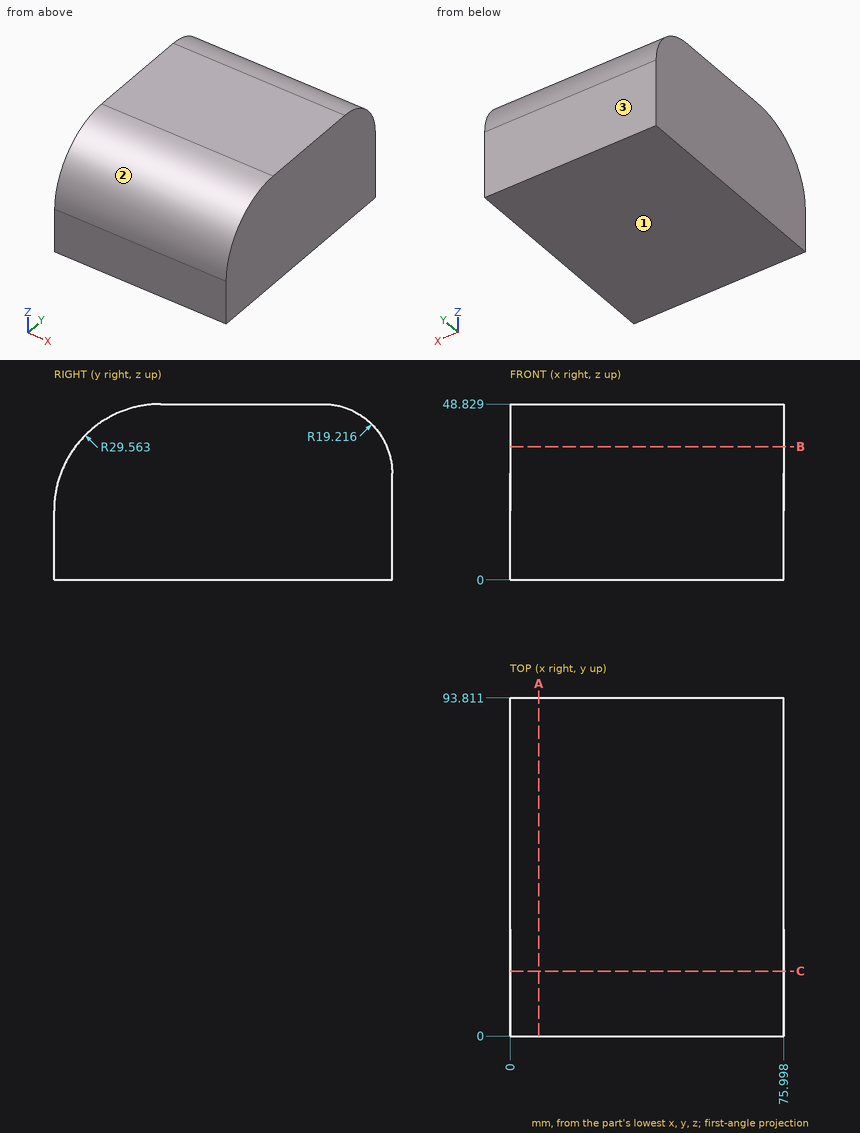
Input: dimensioned drawing with shaded views. Units: mm. Origin: part minimum x, y, z. Give positions to 0.01 mm unless a question says otherwise; leave off trailing zeros. Write each loop counter-clockwise with the first axis right and the second up, starting at its lowest first coordinate (ties: lowest second). Pieces come first, ordered by that corner, then holes. Notation, with made-up numbers: M 85,-28.75 L 133,-28.75 A7 cw 133,-22.75 Z; hole C 74.5,14.25 d4. An arc over 180 degrees is marked long. Write item = value, one per line. Start each with the question number.
1) Cut plane B-B on z = 37. Return the cut outline in (x, y) (1 decimal), then the cut area to 3 significant figures.
2) Cut plane A-A on x = 8. Return the cut outline in (y, z) (1 decimal), then the cut area to 3 significant figures.
3) Draft query along Z for the marked faces 1, 2 and 3. Return one class per face: +Z half, -Z half, draft (parallel to the pull), parting line (faces both ways), or undercut.
4) Cut plane C-C on y = 18. Return the cut outline in (x, z) (1 decimal), then the cut area to 3 significant figures.
5) Material intervals for line 1 along Y through (x, z) = (30.5, 19.5); line 2 along Y through (x, z) = (55.5, 46) (1 decimal); line 3 along Z through (x, y) = (44, 23), sorted ascending. Write a range as [from, to].
6) First-contact query: pin 1 Ø5 at (x, z) = (61.5, 30) entering from -Y; pin 2 Ø10 at (x, y) = (36.5, 54.5) entering from -Z. Flat tips, straight axial feed; report the tip coordinate or a pass-through.
Solved:
q1.outline = M 0,5.9 L 76,5.9 L 76,92.3 L 0,92.3 Z
q1.area = 6,570 mm2
q2.outline = M 0,0 L 93.8,0 L 93.8,29.6 A19.2 ccw 74.6,48.8 L 29.6,48.8 A29.6 ccw 0,19.3 Z
q2.area = 4,310 mm2
q3.face_1 = -Z half
q3.face_2 = +Z half
q3.face_3 = draft
q4.outline = M 0,0 L 76,0 L 76,46.5 L 0,46.5 Z
q4.area = 3,530 mm2
q5.line_1 = [0, 93.81]
q5.line_2 = [16.9, 84.6]
q5.line_3 = [0, 48.09]
q6.pin_1 = 1.17
q6.pin_2 = 0
